from build123d import *

# Parameters (mm, degrees)
SKETCH_1_W      = 300
SKETCH_1_H      = 200
EXTRUDE_1_DEPTH = 80
EXTRUDE_1_DRAFT = -15
SHELL_1_T       = -3
FILLET_1_R      = 10


with BuildPart() as part:
    # 草图1 → 凸台-拉伸1 (with draft: the straight prism first)
    with BuildSketch(Plane.XY):
        Rectangle(SKETCH_1_W, SKETCH_1_H)
    extrude(amount=EXTRUDE_1_DEPTH)
    # 凸台-拉伸1: the draft: its side faces are tilted about the plane it starts from
    extrude_1_sides = [part.faces().sort_by_distance(p)[0] for p in [
        (0, -100, 40),
        (150, 0, 40),
        (0, 100, 40),
        (-150, 0, 40),
    ]]
    draft(extrude_1_sides, Plane.XY, EXTRUDE_1_DRAFT)

    # 抽壳1
    shell_1_openings = [part.faces().sort_by_distance(p)[0] for p in [
        (0, 0, 80),
    ]]
    offset(amount=SHELL_1_T, openings=shell_1_openings, kind=Kind.INTERSECTION)

    # 圆角1
    fillet_1_edges = [part.edges().sort_by_distance(p)[0] for p in [
        (158.014062945, -108.014062945, 41.5),
        (158.014062945, 108.014062945, 41.5),
        (-158.014062945, 108.014062945, 41.5),
        (-158.014062945, -108.014062945, 41.5),
        (160.717967697, -110.717967697, 40),
        (-160.717967697, -110.717967697, 40),
        (-160.717967697, 110.717967697, 40),
        (160.717967697, 110.717967697, 40),
    ]]
    fillet(fillet_1_edges, radius=FILLET_1_R)


solid = part.part
Geometry check sheet. Reference: the model listing, model coordinates, mm. A direction names the side the tool comes from. Give positions to 0.01 mm unless a question says otherwise; leave off trailing zeros. Order: outer loops, then holes, each group sorted by start corner. A loop starts at its lowest first (then second) coordinate and runs counter-clockwise, first axis right, second up. Notation, with made-up numbers: M -35,-3 L 19,-3 A22 ccw 19,12 Z; hole C -14,-30 d9. An arc over 180 degrees is marked long. Use a Markdown table: item, result.
Item 1: Tool access check on faces 4 (the flat face through (-2, 1, 0)), 5 (the cylindrical face through (155.05, 104.9, 40.58)). Record the directions out of +Z, -Z, +X, -X, +Y, -Y that give a thin tool (end or side, any length) a straight path to the whole face; none if there is none.
Answers follow:
| item | result |
|---|---|
| face 4 | -Z, +X, -X, +Y, -Y |
| face 5 | +Z |
Item 2: Section check A-A (x = -102). Record the cut outline in (y, z).
Answers follow:
| item | result |
|---|---|
| outline | M -121.44,80 L -100,0 L 100,0 L 121.44,80 L 118.33,80 L 97.7,3 L -97.7,3 L -118.33,80 Z |
Item 3: Depth check by flat-ended pin: P1, Ø5, axis at x = -32, y = 76, coming from the +Z side; P2, Ø5, axis at y = -33.5, z = 15.5, coming from the +X side; P3, Ø5, axis at x = 79.5, z = 33.5, coming from the +Y side. Enter the tip coordinate at first touch or a pass-through.
Answers follow:
| item | result |
|---|---|
| P1 | stops at z = 3 |
| P2 | stops at x = 154.82 |
| P3 | stops at y = 109.65 |
Item 4: Draft check along X on faces 1 (the cylindrical face through (-158.053, 107.905, 40.196)), 2 (the cylindrical face through (-155.05, 104.9, 40.58)), 3 (the cylindrical face through (157.905, -108.053, 40.196)). Enter one of: +X half, -X half, draft (parallel to the pull), parting line (faces both ways), or undercut.
Answers follow:
| item | result |
|---|---|
| face 1 | -X half |
| face 2 | undercut |
| face 3 | +X half |
Item 5: Section check B-B (y = 15). Record the cut outline in (x, z), and give its area (3 significant figures).
Answers follow:
| item | result |
|---|---|
| outline | M -171.44,80 L -150,0 L 150,0 L 171.44,80 L 168.33,80 L 147.7,3 L -147.7,3 L -168.33,80 Z |
| area | 1,380 mm2 |
Item 6: Material ranges on line 1 along Z through (x, y) = (-51, -93); line 2 along Y through (x, z) = (-103.5, 60); line 3 along X through (y, z) = (51.5, 10), recorded low to high.
Answers follow:
| item | result |
|---|---|
| line 1 | z = 0 to 3 |
| line 2 | y = -116.08 to -112.97, 112.97 to 116.08 |
| line 3 | x = -152.68 to -149.57, 149.57 to 152.68 |
